Can you work these out from the model? Positions are in its coordinate system, mm. A direction names the side the tool comes from. Coordinates: 2 decimals unless noted, no trailing zeros. Order: outer loops, then holes, each group sorted by start corner. A loop starts at its lowest first (then second) coordinate and runs counter-clockwise, first axis right, second up. Notation, with made-up numbers: (71.25, 84.5) -> (96.25, 84.5) arc R21 cw to (96.25, 119.5) -> close; hole circle Ø9 at (-34.5, 2). An arc over 180 degrees is marked (long way). Answer in a Markdown table with one row per item.
```python
from build123d import *

# Parameters (mm, degrees)
F0_R      = 3.17
F0_R_2    = 1.57
F1_DEPTH  = 9.2
F2_R      = 6.07
F2_R_2    = 3.17
F3_DEPTH  = 2.7
F5_DEPTH  = 4
F6_R      = 19.8
F6_R_2    = 12.1
F7_DEPTH  = 8.5
F8_DEPTH  = 4.7
F9_R      = 3.1620005376
F10_DEPTH = 8.5
F11_DEPTH = 3


with BuildPart() as f1:
    # F0 (on Front) → F1 (new body)
    with BuildSketch(Plane.XZ):
        with Locations((-14.4947133958, -5.8518843725)):
            Circle(F0_R)
        with Locations((-14.4947133958, -5.8518843725)):
            Circle(F0_R_2, mode=Mode.SUBTRACT)
    extrude(amount=F1_DEPTH)

    # F8 (add): a face of the model
    f8_faces = [f1.faces().sort_by_distance(p)[0] for p in [
        (-17.575052256, 0, -5.8518843725),
    ]]
    extrude(f8_faces, amount=F8_DEPTH)

    # F9 (on face) → F10 (join, through all)
    with BuildSketch(Plane.XZ.offset(9.2)):
        with Locations((-14.4947133958, -5.8518843725)):
            Circle(F9_R)
    extrude(amount=F10_DEPTH)

    # F11 (add): a face of the model
    f11_faces = [f1.faces().sort_by_distance(p)[0] for p in [
        (-14.4947133958, -17.7, -5.8518843725),
    ]]


with BuildPart() as f3:
    # F2 (on face) → F3 (new body)
    with BuildSketch(Plane.XZ.offset(9.2)):
        with Locations((-14.4947133958, -5.8518843725)):
            Circle(F2_R)
        with Locations((-14.4947133958, -5.8518843725)):
            Circle(F2_R_2, mode=Mode.SUBTRACT)
    extrude(amount=-F3_DEPTH)


with BuildPart() as f5:
    # F4 (on face) → F5 (new body)
    with BuildSketch(Plane.XZ.offset(9.2)):
        with BuildLine():
            Line((-15.9479831574, 6.2612492848), (-15.9479831574, 0.0415787011))
            ThreePointArc((-15.9479831574, 0.0415787011), (-14.5494593079, 0.2178687431), (-13.1479831574, 0.0668331967))
            Line((-13.1479831574, 0.0668331967), (-13.1479831574, 6.2735565541))
            ThreePointArc((-13.1479831574, 6.2735565541), (-14.5483374083, 6.3479977771), (-15.9479831574, 6.2612492848))
        make_face()
    extrude(amount=-F5_DEPTH)


with BuildPart() as f5b:
    # F4 (on face) → F5, piece 2 (new body)
    with BuildSketch(Plane.XZ.offset(9.2)):
        with BuildLine():
            ThreePointArc((-9.3973258546, -2.5561992761), (-10.3108067194, -1.4541775926), (-11.4569494327, -0.5967069155))
            Line((-11.4569494327, -0.5967069155), (-11.6216113174, -0.7184141217))
            ThreePointArc((-11.6216113174, -0.7184141217), (-10.465246014, -1.5657876648), (-9.5481790309, -2.6676999957))
            Line((-9.5481790309, -2.6676999957), (-9.3973258546, -2.5561992761))
        make_face()
        with BuildLine():
            Line((-6.3175093497, 3.2020282617), (-11.4569494327, -0.5967069155))
            ThreePointArc((-11.4569494327, -0.5967069155), (-10.3108067194, -1.4541775926), (-9.3973258546, -2.5561992761))
            Line((-9.3973258546, -2.5561992761), (-4.4629317782, 1.0909794152))
            ThreePointArc((-4.4629317782, 1.0909794152), (-5.3292389654, 2.200076784), (-6.3175093497, 3.2020282617))
        make_face()
    extrude(amount=-F5_DEPTH)


with BuildPart() as f5c:
    # F4 (on face) → F5, piece 3 (new body)
    with BuildSketch(Plane.XZ.offset(9.2)):
        with BuildLine():
            ThreePointArc((-9.0762949538, -8.5878744286), (-9.8553405144, -9.7661045078), (-10.8856064508, -10.7323809722))
            Line((-10.8856064508, -10.7323809722), (-5.8464618601, -14.4569843356))
            ThreePointArc((-5.8464618601, -14.4569843356), (-4.9156940174, -13.4071730995), (-4.1116102126, -12.2574419818))
            Line((-4.1116102126, -12.2574419818), (-9.0762949538, -8.5878744286))
        make_face()
        with BuildLine():
            Line((-11.0433104475, -10.6158165779), (-10.8856064508, -10.7323809722))
            ThreePointArc((-10.8856064508, -10.7323809722), (-9.8553405144, -9.7661045078), (-9.0762949538, -8.5878744286))
            Line((-9.0762949538, -8.5878744286), (-9.2290879071, -8.4749399537))
            ThreePointArc((-9.2290879071, -8.4749399537), (-10.0066754756, -9.6551392938), (-11.0433104475, -10.6158165779))
        make_face()
    extrude(amount=-F5_DEPTH)


with BuildPart() as f5d:
    # F4 (on face) → F5, piece 4 (new body)
    with BuildSketch(Plane.XZ.offset(9.2)):
        with BuildLine():
            ThreePointArc((-13.1479831574, -11.7706019418), (-14.5494593079, -11.9216374882), (-15.9479831574, -11.7453474462))
            Line((-15.9479831574, -11.7453474462), (-15.9479831574, -17.9650180299))
            ThreePointArc((-15.9479831574, -17.9650180299), (-14.5483374083, -18.0517665222), (-13.1479831574, -17.9773252992))
            Line((-13.1479831574, -17.9773252992), (-13.1479831574, -11.7706019418))
        make_face()
    extrude(amount=-F5_DEPTH)


with BuildPart() as f5e:
    # F4 (on face) → F5, piece 5 (new body)
    with BuildSketch(Plane.XZ.offset(9.2)):
        with BuildLine():
            Line((-18.7000286708, -1.4746451241), (-23.6647134121, 2.1949224291))
            ThreePointArc((-23.6647134121, 2.1949224291), (-24.5279332831, 1.0889007916), (-25.2584622432, -0.1089138213))
            Line((-25.2584622432, -0.1089138213), (-20.2193176525, -3.8335171848))
            ThreePointArc((-20.2193176525, -3.8335171848), (-19.5978393815, -2.5650918366), (-18.7000286708, -1.4746451241))
        make_face()
    extrude(amount=-F5_DEPTH)


with BuildPart() as f5f:
    # F4 (on face) → F5, piece 6 (new body)
    with BuildSketch(Plane.XZ.offset(9.2)):
        with BuildLine():
            ThreePointArc((-19.1409038648, -9.7580095787), (-19.9264174704, -8.5614029362), (-20.4098807653, -7.214123335))
            Line((-20.4098807653, -7.214123335), (-25.5493208484, -11.0128585122))
            ThreePointArc((-25.5493208484, -11.0128585122), (-24.8814163191, -12.2516033027), (-24.0752979412, -13.4051882701))
            Line((-24.0752979412, -13.4051882701), (-19.1409038648, -9.7580095787))
        make_face()
        with BuildLine():
            Line((-20.2452188807, -7.0924161289), (-20.4098807653, -7.214123335))
            ThreePointArc((-20.4098807653, -7.214123335), (-19.9264174704, -8.5614029362), (-19.1409038648, -9.7580095787))
            Line((-19.1409038648, -9.7580095787), (-18.9900506885, -9.6465088591))
            ThreePointArc((-18.9900506885, -9.6465088591), (-19.774407608, -8.4465060011), (-20.2452188807, -7.0924161289))
        make_face()
    extrude(amount=-F5_DEPTH)


with BuildPart() as f7:
    # F6 (on face) → F7 (new body, symmetric)
    with BuildSketch(Plane.XZ.offset(9.2)):
        with Locations((-14.4947133958, -5.8518843725)):
            Circle(F6_R)
        with Locations((-14.4947133958, -5.8518843725)):
            Circle(F6_R_2, mode=Mode.SUBTRACT)
    extrude(amount=F7_DEPTH, both=True)


with BuildPart() as f1_1:
    add(f1.part)

    add(f3.part)  # F11 merges F3

    add(f5.part)  # F11 merges F5

    add(f5b.part)  # F11 merges F5b

    add(f5c.part)  # F11 merges F5c

    add(f5d.part)  # F11 merges F5d

    add(f5e.part)  # F11 merges F5e

    add(f5f.part)  # F11 merges F5f

    add(f7.part)  # F11 merges F7
    extrude(f11_faces, amount=-F11_DEPTH)


solid = f1_1.part
```
(1) Suppose I cut it at D-D (y = -8.25). Please give me the cut outline in (x, z).
Response values:
| item | result |
|---|---|
| outline | circle Ø39.6 at (-14.49, -5.85); hole (-25.47, -10.95) -> (-20.41, -7.21) arc R6.07 cw to (-20.22, -3.83) -> (-25.18, -0.17) arc R12.1 ccw to start; hole (-23.99, -13.35) arc R12.1 ccw to (-15.95, -17.86) -> (-15.95, -11.75) arc R6.07 cw to (-19.14, -9.76) -> close; hole (-23.58, 2.14) -> (-18.7, -1.47) arc R6.07 cw to (-15.95, 0.04) -> (-15.95, 6.16) arc R12.1 ccw to start; hole circle Ø3.14 at (-14.49, -5.85); hole (-13.15, -17.88) arc R12.1 ccw to (-5.93, -14.4) -> (-10.89, -10.73) arc R6.07 cw to (-13.15, -11.77) -> close; hole (-13.15, 0.07) arc R6.07 cw to (-11.46, -0.6) -> (-6.4, 3.14) arc R12.1 ccw to (-13.15, 6.17) -> close; hole (-9.4, -2.56) arc R6.07 cw to (-9.08, -8.59) -> (-4.19, -12.2) arc R12.1 ccw to (-4.54, 1.03) -> close |
(2) We'd pull the mould along Z, two halves only. Please class faces 1 (the flat face through (-15, -9.2, -6)), 2 (the flat face through (-15.948, -7, -15)), 3 (the flat face through (-16, 4.7, -7)): +Z half, -Z half, draft (parallel to the pull), parting line (faces both ways), or undercut.
Response values:
| item | result |
|---|---|
| face 1 | undercut |
| face 2 | undercut |
| face 3 | draft |
(3) Will these pins go through, and if not, where does the flat tip stop? pin 1 Ø20 at (x, z) = (-24, -13.5) entering from +Y; pin 2 Ø10 at (x, z) = (-27, -9.5) entering from +Y; pin 3 Ø3 at (y, z) = (-7.5, 3.5) entering from +X; pin 4 Ø2 at (y, z) = (-7, -15) entering from -X.
Response values:
| item | result |
|---|---|
| pin 1 | y = 4.7 |
| pin 2 | y = -0.7 |
| pin 3 | x = 3.68 |
| pin 4 | x = -32.54 |
(4) On a 3-axis mill with a long thin cutter (end or side, diameter ignored), from which of +Z, -Z, +X, -X, +Y, -Y can I reach the whole of each face in a straight line? I mean faces 4 (the cylindrical face through (-10.48, -5.86, -1.55)), 5 (the flat face through (-15.948, -7, 3)), 6 (the flat face through (-15, -17.7, -6)), 7 (the flat face through (-16.5, -9.2, -8.5)). Say none if no direction works.
Response values:
| item | result |
|---|---|
| face 4 | +Y |
| face 5 | +Y, -Y |
| face 6 | +Z, -Z, +X, -X, -Y |
| face 7 | -Y |
(5) Suppose I cut it at C-C (z = 4). Please give me the cut outline in (x, y).
Response values:
| item | result |
|---|---|
| outline | (-31.67, -17.7) -> (-21.52, -17.7) -> (-21.52, -0.7) -> (-31.67, -0.7) -> close; (-15.95, -9.2) -> (-13.15, -9.2) -> (-13.15, -5.2) -> (-15.95, -5.2) -> close; (-7.47, -17.7) -> (2.68, -17.7) -> (2.68, -0.7) -> (-7.47, -0.7) -> close |
(6) Suppose I cut it at A-A (y = -6). Please give me the cut outline in (x, z).
Response values:
| item | result |
|---|---|
| outline | circle Ø39.6 at (-14.49, -5.85); circle Ø6.34 at (-14.49, -5.85); hole (-25.47, -10.95) -> (-20.25, -7.09) arc R5.88 ccw to (-18.99, -9.65) -> (-23.99, -13.35) arc R12.1 ccw to (-15.95, -17.86) -> (-15.95, -11.75) arc R6.07 ccw to (-13.15, -11.77) -> (-13.15, -17.88) arc R12.1 ccw to (-5.93, -14.4) -> (-11.04, -10.62) arc R5.88 ccw to (-9.23, -8.47) -> (-4.19, -12.2) arc R12.1 ccw to (-4.54, 1.03) -> (-9.55, -2.67) arc R5.88 ccw to (-11.62, -0.72) -> (-6.4, 3.14) arc R12.1 ccw to (-13.15, 6.17) -> (-13.15, 0.07) arc R6.07 ccw to (-15.95, 0.04) -> (-15.95, 6.16) arc R12.1 ccw to (-23.58, 2.14) -> (-18.7, -1.47) arc R6.07 ccw to (-20.22, -3.83) -> (-25.18, -0.17) arc R12.1 ccw to start; hole circle Ø3.14 at (-14.49, -5.85) |
(7) Suppose I cut it at B-B (x = -22). Please give me the cut outline in (y, z), and give its area (3 significant figures).
Response values:
| item | result |
|---|---|
| outline | (-17.7, -24.17) -> (-0.7, -24.17) -> (-0.7, -15.34) -> (-17.7, -15.34) -> close; (-17.7, 3.64) -> (-0.7, 3.64) -> (-0.7, 12.47) -> (-17.7, 12.47) -> close; (-9.2, -11.87) -> (-5.2, -11.87) -> (-5.2, -8.39) -> (-9.2, -8.39) -> close; (-9.2, -2.52) -> (-5.2, -2.52) -> (-5.2, 0.96) -> (-9.2, 0.96) -> close |
| area | 328 mm2 |
(8) I need wall thicknesses on line 1 (X direction, y = -15, z = -3); line 2 (X direction, y = -13.5, z = -5.5); line 3 (Y direction, x = -12.5, z = 11). Which ranges of each line are inside material? Lowest first, please. Write a range as [from, to].
Response values:
| item | result |
|---|---|
| line 1 | [-34.09, -26.25], [-15.86, -13.13], [-2.74, 5.1] |
| line 2 | [-34.29, -26.59], [-17.64, -11.35], [-2.4, 5.3] |
| line 3 | [-17.7, -0.7] |
